```python
from build123d import *

# Parameters (mm, degrees)
F0_W          = 40
F0_H          = 50
F1_DEPTH      = 50
F2_W          = 25
F2_H          = 25
F3_DEPTH      = 139.9
F3_DEPTH_BACK = 82.6
F5_W          = 20
F5_H          = 50
F6_DEPTH      = 5
F7_START      = -45
F7_DEPTH      = 30.1


with BuildPart() as f1:
    # F0 (on Front) → F1 (new body)
    with BuildSketch(Plane.XZ):
        with Locations((20, 25)):
            Rectangle(F0_W, F0_H)
    extrude(amount=-F1_DEPTH)


with BuildPart() as f3:
    # F2 (on face) → F3 (new body, two sides)
    with BuildSketch(Plane.YZ.offset(40)) as f3_sk:
        with Locations((25, 25)):
            Rectangle(F2_W, F2_H)
    extrude(amount=-F3_DEPTH)
    extrude(f3_sk.sketch, amount=F3_DEPTH_BACK)


with BuildPart() as f1_1:
    add(f1.part)

    # F4: cut F3
    add(f3.part, mode=Mode.SUBTRACT)

    # F5 (on face) → F6 (cut)
    with BuildSketch(Plane.XY.offset(50)):
        with Locations((20, 25)):
            Rectangle(F5_W, F5_H)
    extrude(amount=-F6_DEPTH, mode=Mode.SUBTRACT)

    # F5 (on face) → F7 (cut)
    with BuildSketch(Plane.XY.offset(50).offset(F7_START)):
        with Locations((20, 25)):
            Rectangle(F5_W, F5_H)
    extrude(amount=-F7_DEPTH, mode=Mode.SUBTRACT)


solid = f1_1.part
```
CAD build for the part. Positions are in the model's coordinates, mm. A direction names the side the tool comes from. Coordinates: 2 decimals unless noted, no trailing zeros. Order: outer loops, then holes, each group sorted by start corner. A loop starts at its lowest first (then second) coordinate and runs counter-clockwise, first axis right, second up. Notation, with made-up numbers: (-27.5, -0.75) - (-4.5, -0.75) arc R36 cw to (-4.5, 38.25) - close; hole circle Ø9 at (1, 15). An arc over 180 degrees is marked (long way). Use a Markdown table: item, result. Add a question column.
(1) Saw through at C-C (x = 32). Give the cut face in (y, z).
(2) Saw through at B-B (y = 32.5). Give the cut face in (x, z), then the cut area to 3 significant figures.
(3) Saw through at A-A (z = 32). Give the cut face in (x, y), then the cut area to 3 significant figures.
(4) Saw through at D-D (y = 7.5). Give the cut face in (x, z).
(5) Which spindle directions (+Z, -Z, +X, -X, +Y, -Y) get a long thin tool onto all of the face, cutting with end or side? Do faces 4 (the face through (30, 25, 3)), 5 (the face through (30, 25, 48)), 6 (the face through (35, 25, 50)), 7 (the face through (20, 25, 12.5)). Say none if no direction does.
(6) Drill centre lines: line 1 along X through (y, z) = (46, 4.5); line 2 along Y through (x, z) = (9, 26); line 3 along Z through (x, y) = (10.5, 25). Where is each one in solid material? Low to high. Write a range as [from, to].
(7) Pull direction Y, two halves, no side cores. Call faces 1 (the face through (10, 25, 3)), 2 (the face through (20, 50, 25)), 3 (the face through (20, 25, 37.5)): +Y half, -Y half, draft (parallel to the pull), parting line (faces both ways), or undercut.
(8) Flat gauge pin, fed straight in: pin 1 (5 mm diameter, centred on x = 18.5, y = 15.5, fed in from -Z). Where does the tip first touch, or does it go through?
Solved:
| question | item | result |
|---|---|---|
| 1 | outline | (0, 0) - (50, 0) - (50, 50) - (0, 50) - close; hole (12.5, 12.5) - (37.5, 12.5) - (37.5, 37.5) - (12.5, 37.5) - close |
| 2 | outline | (0, 0) - (10, 0) - (10, 5) - (30, 5) - (30, 0) - (40, 0) - (40, 12.5) - (0, 12.5) - close; (0, 37.5) - (40, 37.5) - (40, 50) - (30, 50) - (30, 45) - (10, 45) - (10, 50) - (0, 50) - close |
| 2 | area | 800 mm² |
| 3 | outline | (0, 0) - (40, 0) - (40, 12.5) - (0, 12.5) - close; (0, 37.5) - (40, 37.5) - (40, 50) - (0, 50) - close |
| 3 | area | 1,000 mm² |
| 4 | outline | (0, 0) - (10, 0) - (10, 5) - (30, 5) - (30, 0) - (40, 0) - (40, 50) - (30, 50) - (30, 45) - (10, 45) - (10, 50) - (0, 50) - close |
| 5 | face 4 | -Z, +Y, -Y |
| 5 | face 5 | +Z, +Y, -Y |
| 5 | face 6 | +Z, +X, -X, +Y, -Y |
| 5 | face 7 | +X, -X |
| 6 | line 1 | x = [0, 10], [30, 40] |
| 6 | line 2 | y = [0, 12.5], [37.5, 50] |
| 6 | line 3 | z = [5, 12.5], [37.5, 45] |
| 7 | face 1 | draft |
| 7 | face 2 | +Y half |
| 7 | face 3 | undercut |
| 8 | pin 1 | stops at z = 5 |
